from build123d import *

# Parameters (mm, degrees)
SKETCH1_W           = 61.345012487
SKETCH1_H           = 38.657423861
BOSS_EXTRUDE1_DEPTH = 10
BOSS_EXTRUDE2_DEPTH = 10
SKETCH3_W           = 55.653219253
SKETCH3_H           = 4.667772156
BOSS_EXTRUDE3_DEPTH = 3
BOSS_EXTRUDE4_DEPTH = 3


with BuildPart() as part:
    # Sketch1 → Boss-Extrude1 (new body)
    with BuildSketch(Plane.XY):
        with Locations((-23.425520154, 10.330558338)):
            Rectangle(SKETCH1_W, SKETCH1_H)
    extrude(amount=BOSS_EXTRUDE1_DEPTH)

    # Sketch2 → Boss-Extrude2 (add)
    with BuildSketch(Plane(origin=(-8.887322321, 1.300253896, 19.221447103), x_dir=(0.908038086, 0.028271458, 0.417932481), z_dir=(-0.418887615, 0.061285079, 0.905967607))):
        Polygon((-87.68448092, 45.888055238), (-37.545380932, 30.082102221), (-37.545380932, -9.327101998), (-109.421725422, 13.33134469), align=None)
    extrude(amount=BOSS_EXTRUDE2_DEPTH)

    # Sketch3 → Boss-Extrude3 (add)
    with BuildSketch(Plane.XZ):
        with Locations((-25.061108276, -1.221803115)):
            Rectangle(SKETCH3_W, SKETCH3_H)
    extrude(amount=BOSS_EXTRUDE3_DEPTH)

    # Sketch5 → Boss-Extrude4 (add)
    with BuildSketch(Plane(origin=(-3.775073918, -13.275413408, -0.84743311), x_dir=(0.962011868, -0.272453087, -0.017391983), z_dir=(-0.27300763, -0.960057797, -0.061285079))):
        Polygon((-47.103632436, 2.289571082), (-100.846305257, -21.775814591), (-98.638237359, -26.887445035), (-46.85648275, -2.542586037), (-46.85648275, 2.289571082), align=None)
    extrude(amount=BOSS_EXTRUDE4_DEPTH)


solid = part.part
Verification items for the finished model (mm, model axes). A direction names the side the tool comes from. Coordinates: 2 decimals unless noted, no trailing zeros. Order: outer loops, then holes, each group sorted by start corner. A loop starts at its lowest first (then second) coordinate and runs counter-clockwise, first axis right, second up. Notation, with made-up numbers: M 2,-24.5 L 9,-24.5 A21 cw 9,-20.5 Z; hole C 48.25,34 d7. An arc over 180 degrees is marked long. Write each question's results on one line, items separated by ' | '.
1) Section check A-A on x = -28.5. Record the cut outline in (y, z).
Solved:
outline: M -9,0 L -3,0 L -3,-3.56 L 0,-3.56 L 0,0 L 29.66,0 L 29.66,10 L -9,10 Z
2) Section check C-C on y = 10. Record the cut outline in (x, z), plus the area to 3 significant figures.
Solved:
outline: M -105.71,-15.1 L -103.46,-25.1 L -92.33,-19.95 L -91.75,-22.52 L -81.77,-18.03 L -82.37,-15.34 L -49.19,0 L 7.25,0 L 7.25,10 L -46.26,10 L -47.17,11.97 L -51.43,10 L -54.1,10 L -54.1,8.77 Z | area: 1,210 mm²
3) Access from +Z, -Z, +X, -X, +Y, -Y to the whole of each face (thin tool, end or side, straight path). Record for faces 1 (the face through (2.766, -1, -2)), 2 (the face through (-99.55, 13.95, -24.9)), 3 (the face through (-48.547, -7.948, 11.431)).
Solved:
face 1: -Z, +X, +Y, -Y | face 2: -Z | face 3: -X, -Y
4) Section check D-D on z = -14. Record the cut outline in (x, y), plus the area to 3 significant figures.
Solved:
outline: M -103.44,9.29 L -80.52,2.77 L -80.03,6.12 L -73.62,4.3 L -73.19,7.3 L -79.59,9.12 L -75.02,40.35 L -91.52,45.05 L -99.97,33.02 Z | area: 871 mm²
5) Section check B-B on z = -6. Record the cut outline in (x, y).
Solved:
outline: M -86.9,4.07 L -63.98,-2.45 L -63.49,0.91 L -56.58,-1.05 L -56.16,1.95 L -63.05,3.91 L -58.49,35.14 L -81.4,41.66 Z
6) Gauge pin test, flat ends, axial feed: pin 1 Ø1.5 at (y, z) = (26, 3.5) entering from -X; pin 2 Ø2.5 at (x, y) = (-38.5, -1) entering from -Z; pin 3 Ø11 at (y, z) = (5, 7) entering from -X. Record the tip position at first contact, or that the pin passes through.
Solved:
pin 1: stops at x = -64.77 | pin 2: stops at z = -3.56 | pin 3: stops at x = -70.57
7) Scan lines: line 1 along Z through (x, y) = (-32, 26.5); line 2 along Y through (x, z) = (-21, 1.5); line 3 along X through (y, z) = (-3, 7.5). Record each from-to range of solid material in increasing order. Write a range as [from, to].
Solved:
line 1: z = [0, 10] | line 2: y = [-9, 29.66] | line 3: x = [-58.74, 7.25]
8) Release check for a two-part mould opening along Z. For faces 4 (the face through (-76.02, 4.95, -13.45)), 5 (the face through (-73.06, 7.2, -12.95)), 6 (the face through (-68.13, 37.83, -5.2)) record: pulls with the +Z half, pulls with the -Z half, needs draft (parallel to the pull), parting line crosses it, or undercut.
Solved:
face 4: pulls with the -Z half | face 5: undercut | face 6: pulls with the +Z half
